Answer from the drawing. Dimensions are ordinates in mm from the lowest x, y and z of the part. A direction names the side the tool comes from. Round coordinates to 2 decimals unless told otherwise and drop trailing zeros. Order: outer loops, then holes, each group sorted by start corner. A loop starts at its lowest first (then second) coordinate and runs counter-clockwise, first axis right, second up. Notation, with made-up numbers: M 89,29.5 L 118,29.5 A19 cw 118,53.5 Z; hole C 31.25,-29.75 d6. An arc over 180 degrees is marked long. Write item = value, one per line. Start each with the question number.
(1) Which of the six approach directions +Z, -Z, +X, -X, +Y, -Y give full straight-line access (tool end or side, diameter ignored) to the marked faces 5, 6 and 7?
(2) A cutting plane is placed at A-A, the plane y = 0.6. Count the separate pieces of the cut face and the enclosed holes in it, and give its area (3 significant figures).
(3) A cutting plane is placed at D-D, the plane z = 18. Determine the outline of the cut face in (x, y) (1 decimal).
(4) Each of these flat-tipped pins is pushed along its axis until it touches: pin 1 (1.2 mm diameter, centred on x = 26, y = 3, fed in from +Z); pin 2 (3 mm diameter, centred on x = 2.5, z = 13, fed in from -Y); pin 3 (2.5 mm diameter, centred on x = 24.42, z = 12.5, fed in from -Y); pin 4 (1.2 mm diameter, centred on x = 25.5, y = 1, fed in from -Z). Where does it stop, or does it pass through?
(5) Straight lines are drawn through the part: probe 1 along X at (y, z) = (4.7, 12.5); probe 2 along X at (y, z) = (3.9, 3.75); probe 3 along Z at (x, y) = (2.5, 0.45). For each, find the intervals that lie inside material, in ascending order. Write a range as from..to.
(6) A cutting plane is placed at B-B, the plane z = 12. Determine the outline of the cut face in (x, y).
(7) For a pull along Z with two mould halves and no side action, classify the marked faces 1, 2, 3 and 4 as released by +Z, released by -Z, zero draft, split by the parting line, or undercut.
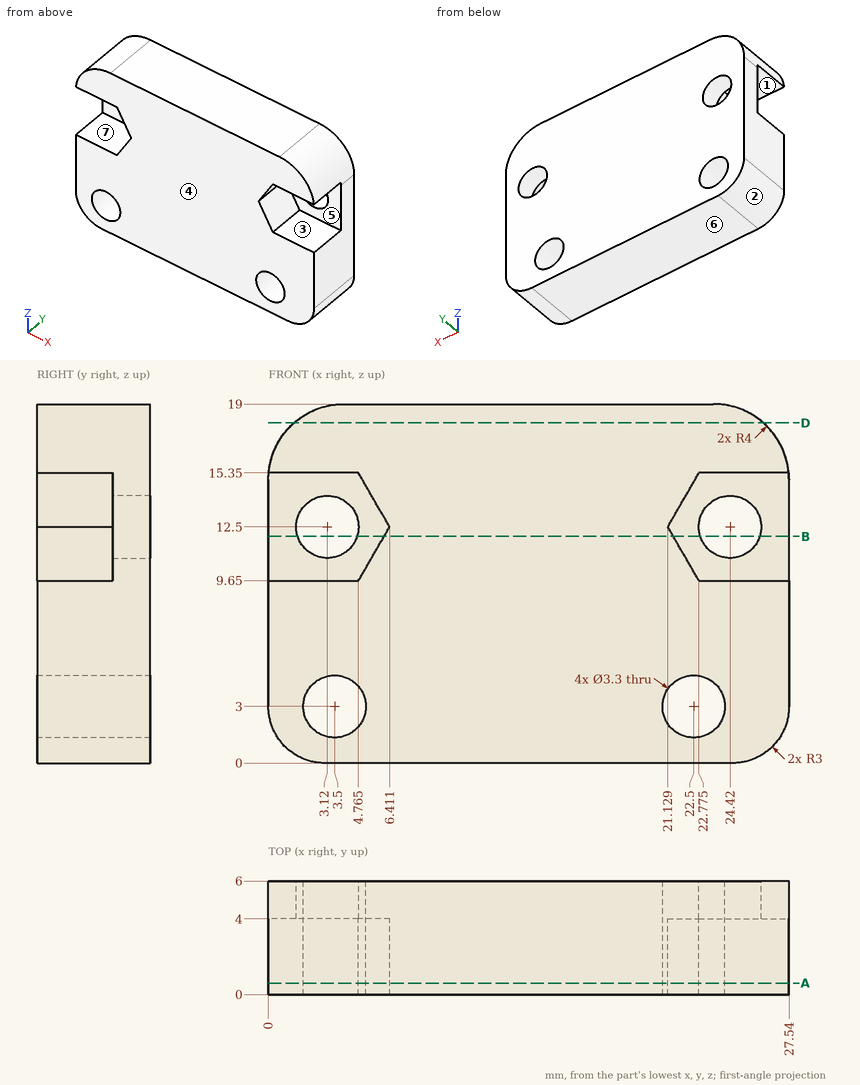
Reported:
q1.face_5 = +X, -Y
q1.face_6 = -Z, +X, -X, +Y, -Y
q1.face_7 = -X, -Y
q2.separate_pieces = 1
q2.enclosed_holes = 2
q2.area = 432 mm²
q3.outline = M 1.4,0 L 26.2,0 L 26.2,6 L 1.4,6 Z
q4.pin_1 = 18.54
q4.pin_2 = 4
q4.pin_3 = through
q4.pin_4 = 0.02
q5.probe_1 = 0..1.47, 4.77..22.77, 26.07..27.54
q5.probe_2 = 0..2.03, 4.97..21.03, 23.97..27.54
q5.probe_3 = 0.04..1.69, 4.31..9.65, 15.35..18.71
q6.outline = M 0,4 L 1.55,4 L 1.55,6 L 0,6 Z; M 4.69,4 L 6.12,4 L 6.12,0 L 21.42,0 L 21.42,4 L 22.85,4 L 22.85,6 L 4.69,6 Z; M 25.99,4 L 27.54,4 L 27.54,6 L 25.99,6 Z
q7.face_1 = undercut
q7.face_2 = released by -Z
q7.face_3 = undercut
q7.face_4 = zero draft
